from build123d import *

# Parameters (mm, degrees)
SKETCH1_W           = 450
SKETCH1_H           = 100
BOSS_EXTRUDE1_DEPTH = 200
SKETCH2_R           = 40
BOSS_EXTRUDE2_DEPTH = 90


with BuildPart() as part:
    # Sketch1 → Boss-Extrude1 (new body)
    with BuildSketch(Plane.XY):
        with Locations((225, 590)):
            Rectangle(SKETCH1_W, SKETCH1_H)
    extrude(amount=BOSS_EXTRUDE1_DEPTH)

    # Sketch2 → Boss-Extrude2 (add)
    with BuildSketch(Plane.XZ.offset(-540)):
        with Locations(Location((80, 100, 0), (0, 0, 90))):
            Circle(SKETCH2_R)
        with Locations(Location((370, 100, 0), (0, 0, 90))):
            Circle(SKETCH2_R)
    extrude(amount=BOSS_EXTRUDE2_DEPTH)


solid = part.part
The listing builds one solid part. Answer for the finished solid, in the listing's coordinates (mm). A direction names the side the tool comes from. Give positions to 0.01 mm unless a question says otherwise; leave off trailing zeros. Order: outer loops, then holes, each group sorted by start corner. A loop starts at its lowest first (then second) coordinate and runs counter-clockwise, first axis right, second up. Notation, with made-up numbers: (47.25, 61.25) -> (58.25, 61.25) arc R10 cw to (58.25, 68.25) -> close; hole circle Ø5 at (76.5, 75). An arc over 180 degrees is marked (long way). Put each result on its own line as item: value.
Item 1: A cutting plane is placed at D-D on z = 177. Give the vertices of the cut face in (x, y), plus the area to 3 significant figures.
Established:
outline: (0, 540) -> (450, 540) -> (450, 640) -> (0, 640) -> close
area: 45,000 mm^2
Item 2: Straight lines are drawn through the part: line 1 (Y direction, x = 139, z = 171); line 2 (X direction, y = 534, z = 137); line 3 (X direction, y = 526.5, z = 117.5). For each, find the intervals that lie inside material, in ascending order.
Established:
line 1: y = 540 to 640
line 2: x = 64.8 to 95.2, 354.8 to 385.2
line 3: x = 44.03 to 115.97, 334.03 to 405.97
Item 3: A cutting plane is placed at A-A on x = 394. Give the vertices of the cut face in (y, z), plus the area to 3 significant figures.
Established:
outline: (450, 68) -> (540, 68) -> (540, 0) -> (640, 0) -> (640, 200) -> (540, 200) -> (540, 132) -> (450, 132) -> close
area: 25,800 mm^2
Item 4: A cutting plane is placed at C-C on z = 100. Give the vertices of the cut face in (x, y).
Established:
outline: (0, 540) -> (40, 540) -> (40, 450) -> (120, 450) -> (120, 540) -> (330, 540) -> (330, 450) -> (410, 450) -> (410, 540) -> (450, 540) -> (450, 640) -> (0, 640) -> close
Item 5: Given P1, Ø1, axis at x = 138.5, z = 165.5, coming from the -Y side; P2, Ø1, axis at x = 77, y = 538.5, coming from the -Z side, each flat-ended and moving along its own axis, determine where each tip first touches the part or whether it passes through.
Established:
P1: stops at y = 540
P2: stops at z = 60.08
Item 6: For faces 1 (the face through (67.985, 495.63, 138.153)), 2 (the face through (222, 591, 0)), determine the directions among +Z, -Z, +X, -X, +Y, -Y from which every point of the face is accessible in a straight line to the end or side of a thin tool.
Established:
face 1: -Y
face 2: -Z, +X, -X, +Y, -Y
Item 7: A cutting plane is placed at B-B on y = 467.5. Give the vertices of the cut face in (x, z), plus the area to 3 significant figures.
Established:
outline: circle Ø80 at (80, 100); circle Ø80 at (370, 100)
area: 10,100 mm^2
Item 8: For a pull along X with two mould halves and no side action, classify faces 3 (the face through (369, 450, 99)), 4 (the face through (0, 589, 99)), 5 (the face through (222, 540, 99)) as released by +X, released by -X, zero draft, split by the parting line, or undercut.
Established:
face 3: zero draft
face 4: released by -X
face 5: undercut
